Verification items for the finished model (mm, model axes). A direction names the side the tool comes from. Round coordinates to 2 decimals unless told otherwise and drop trailing zeros. Answer in a Markdown table with one row per item. Add a question column.
1. Set-up check for faces 1 (the flat face through (-5, -7.5, 106)), 2 (the flat face through (2.65, 0, 106)), 3 (the flat face through (-2.65, 0, 106)): record each of +Z, -Z, +X, -X, +Y, -Y from which the full face is reachable in a straight line by a thin tool's end or side.
2. Go/stop test with flat-tipped pins: pin 1 Ø1.7 at (y, z) = (0.5, 69) entering from +X; pin 2 Ø2 at (x, y) = (0, 0) entering from -Z; pin 3 Ø1 at (x, z) = (1, 140) entering from -Y. Record where each tip stops, or that it passes through.
3. Draft check along X on faces 4 (the flat face through (0, 2.65, 106)), 5 (the flat face through (0, 2, 0)), 6 (the flat face through (-7.5, -5, 106)), 7 (the flat face through (0, -2.65, 106)). Enter one of: pulls with the +X half, pulls with the -X half, needs draft (parallel to the pull), parting line crosses it, or undercut.
4. Material ranges on probe 1 along Y at (x, z) = (7.25, 60.5); probe 2 along Y at (x, z) = (0, 135.5); probe 3 along X at (y, z) = (2.5, 13), recorded low to high.
```python
from build123d import *

# Parameters (mm, degrees)
SKETCH_2_R      = 1.25
EXTRUDE_1_DEPTH = 215


with BuildPart() as part:
    # ｽｹｯﾁ2 → ﾎﾞｽ - 押し出し1 (new body)
    with BuildSketch(Plane.XY):
        Polygon((1.7, 2.65), (-1.7, 2.65), (-2.85, 3.8), (-2.85, 6.4), (-1.7, 6.4), (-1.7, 7.5), (-7.5, 7.5), (-7.5, 1.7), (-6.4, 1.7), (-6.4, 2.85), (-3.8, 2.85), (-2.65, 1.7), (-2.65, -1.7), (-3.8, -2.85), (-6.4, -2.85), (-6.4, -1.7), (-7.5, -1.7), (-7.5, -7.5), (-1.7, -7.5), (-1.7, -6.4), (-2.85, -6.4), (-2.85, -3.8), (-1.7, -2.65), (1.7, -2.65), (2.85, -3.8), (2.85, -6.4), (1.7, -6.4), (1.7, -7.5), (7.5, -7.5), (7.5, -1.7), (6.4, -1.7), (6.4, -2.85), (3.8, -2.85), (2.65, -1.7), (2.65, 1.7), (3.8, 2.85), (6.4, 2.85), (6.4, 1.7), (7.5, 1.7), (7.5, 7.5), (1.7, 7.5), (1.7, 6.4), (2.85, 6.4), (2.85, 3.8), align=None)
        Circle(SKETCH_2_R, mode=Mode.SUBTRACT)
    extrude(amount=EXTRUDE_1_DEPTH)


solid = part.part
```
Geometry check:
| question | item | result |
|---|---|---|
| 1 | face 1 | +Z, -Z, +X, -X, -Y |
| 1 | face 2 | +Z, -Z, +X |
| 1 | face 3 | +Z, -Z, -X |
| 2 | pin 1 | stops at x = 2.65 |
| 2 | pin 2 | passes through |
| 2 | pin 3 | stops at y = -2.65 |
| 3 | face 4 | undercut |
| 3 | face 5 | needs draft |
| 3 | face 6 | pulls with the -X half |
| 3 | face 7 | undercut |
| 4 | probe 1 | y = -7.5 to -1.7, 1.7 to 7.5 |
| 4 | probe 2 | y = -2.65 to -1.25, 1.25 to 2.65 |
| 4 | probe 3 | x = -7.5 to -6.4, -3.45 to 3.45, 6.4 to 7.5 |
